Input: part model. Units: mm. Frame: model coordinates. Face numbers are marked on the shaded views. A direction names the side the tool comes from. Give positions to 0.01 mm unless a question says otherwise; leave off trailing zeros. Loops run counter-clockwise (first coordinate to the right, second up) from the corner with the lowest first, then second, coordinate; pieces in that order, holes last. Notation, with made-up numbers: (-34, 75) - (-7, 75) arc R21 ccw to (-7, 91) - close; hole circle Ø5 at (27.25, 63.5). An arc over 180 degrees is marked (long way). Answer as a JSON object with one key per item and string values. Group by question number.
(1) Access query for the marked faces 5, 6 and 7. Directions: +Z, -Z, +X, -X, +Y, -Y. A direction counts if a zero-diameter tool reaches every point of the face in a straight line with its end or side. Return the directions, or none.
(2) Section query D-D (x = -8). Return loops of the section in (y, z).
(3) Section query C-C (y = 8). Return loops of the section in (x, z).
(4) Pin query (flat end, axial travel): P1, Ø1, axis at x = -2, z = -16.5, coming from the +Y side; P2, Ø12, axis at x = 2.5, y = -5.5, coming from the +Z side; P3, Ø3, axis at x = -7.5, y = -1, coming from the +Z side; P4, Ø8, axis at x = -7, y = 4, coming from the -Z side. Return the tip coordinate at first contact, or that it passes through.
(5) Mould query, pull axis X, two halves, no side actions, for the marked faces 1, 2, 3 and 4. Classes: +X half, -X half, draft (parallel to the pull), parting line (faces both ways), or undercut.
(6) Section query A-A (z = -45.9). Return loops of the section in (x, y) (3 decimals).
(7) Section query B-B (x = 8). Return loops of the section in (y, z), plus the area to 3 significant figures.
(8) Material intervals for L1, parallel to Y at x = 5.25, z = -13.5; L2, parallel to X at y = -9.4, z = -45.9; L3, parallel to Z at x = 1, y = -10.5, sorted ascending.
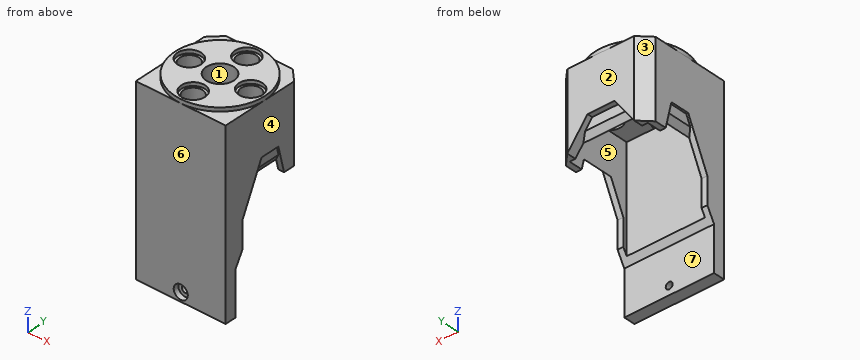
```python
from build123d import *

# Parameters (mm, degrees)
SKETCH_1_R                  = 11.7
EXTRUDE_1_DEPTH             = 7.7
SKETCH_1_3_R                = 2.5
CUT_EXTRUDE_1_DEPTH         = 19.250205478
SKETCH_1_5_R                = 3.1
SKETCH_1_5_R_2              = 2.5
CUT_EXTRUDE_2_DEPTH         = 0.9
CUT_EXTRUDE_START           = -6.8
SKETCH_1_6_R                = 3.1
SKETCH_1_6_R_2              = 2.5
CUT_EXTRUDE_3_DEPTH         = 0.9
EXTRUDE_START               = -7.7
SKETCH_2_W                  = 23.4
SKETCH_2_H                  = 2.4
SKETCH_2_H_2                = 4
EXTRUDE_3_DEPTH             = 40.5
SKETCH_3_W                  = 1.5
SKETCH_3_H                  = 23.4
EXTRUDE_4_DEPTH             = 40.3
EXTRUDE_START_2             = -1
EXTRUDE_5_DEPTH             = 6.7
CUT_EXTRUDE_5_DEPTH         = 55.842410596
CHAMFER_1_SIZE              = 3
CUT_EXTRUDE_6_REACH         = 56.842
EXTRUDE_6_REACH             = 52.961
EXTRUDE_6_DIRECTION_2_REACH = 52.961
EXTRUDE_7_REACH             = 52.961
EXTRUDE_7_DIRECTION_2_REACH = 52.961
HOLE_WIZARD_1_D             = 1.8
HOLE_WIZARD_1_CBORE_D       = 3.67
HOLE_WIZARD_1_CBORE_DEPTH   = 1.35
CUT_EXTRUDE_7_REACH         = 52.961
SKETCH_19_R                 = 3.6


with BuildPart() as part:
    # 草图1 → 凸台-拉伸1 (new body)
    with BuildSketch(Plane.XY):
        Circle(SKETCH_1_R)
    extrude(amount=-EXTRUDE_1_DEPTH)

    # 草图1<3> → 切除-拉伸1 (cut, through all)
    with BuildSketch(Plane.XY):
        with Locations((-8, 0)):
            Circle(SKETCH_1_3_R)
        with Locations((0, 8)):
            Circle(SKETCH_1_3_R)
        with Locations((8, 0)):
            Circle(SKETCH_1_3_R)
        with Locations((0, -8)):
            Circle(SKETCH_1_3_R)
    extrude(amount=-CUT_EXTRUDE_1_DEPTH, mode=Mode.SUBTRACT)

    # 草图1<5> → 切除-拉伸2 (cut)
    # profile 1 of 4: a face of its own
    with BuildSketch(Plane.XY):
        with Locations((-8, 0)):
            Circle(SKETCH_1_5_R)
        with Locations((-8, 0)):
            Circle(SKETCH_1_5_R_2, mode=Mode.SUBTRACT)
    # profile 2 of 4: a face of its own
    with BuildSketch(Plane.XY):
        with Locations((0, 8)):
            Circle(SKETCH_1_5_R)
        with Locations((0, 8)):
            Circle(SKETCH_1_5_R_2, mode=Mode.SUBTRACT)
    # profile 3 of 4: a face of its own
    with BuildSketch(Plane.XY):
        with Locations((8, 0)):
            Circle(SKETCH_1_5_R)
        with Locations((8, 0)):
            Circle(SKETCH_1_5_R_2, mode=Mode.SUBTRACT)
    # profile 4 of 4: a face of its own
    with BuildSketch(Plane.XY):
        with Locations((0, -8)):
            Circle(SKETCH_1_5_R)
        with Locations((0, -8)):
            Circle(SKETCH_1_5_R_2, mode=Mode.SUBTRACT)
    extrude(amount=-CUT_EXTRUDE_2_DEPTH, mode=Mode.SUBTRACT)

    # 草图1<6> → 切除-拉伸3 (cut)
    # profile 1 of 4: a face of its own
    with BuildSketch(Plane.XY.offset(CUT_EXTRUDE_START)):
        with Locations((-8, 0)):
            Circle(SKETCH_1_6_R)
        with Locations((-8, 0)):
            Circle(SKETCH_1_6_R_2, mode=Mode.SUBTRACT)
    # profile 2 of 4: a face of its own
    with BuildSketch(Plane.XY.offset(CUT_EXTRUDE_START)):
        with Locations((8, 0)):
            Circle(SKETCH_1_6_R)
        with Locations((8, 0)):
            Circle(SKETCH_1_6_R_2, mode=Mode.SUBTRACT)
    # profile 3 of 4: a face of its own
    with BuildSketch(Plane.XY.offset(CUT_EXTRUDE_START)):
        with Locations((0, -8)):
            Circle(SKETCH_1_6_R)
        with Locations((0, -8)):
            Circle(SKETCH_1_6_R_2, mode=Mode.SUBTRACT)
    # profile 4 of 4: a face of its own
    with BuildSketch(Plane.XY.offset(CUT_EXTRUDE_START)):
        with Locations((0, 8)):
            Circle(SKETCH_1_6_R)
        with Locations((0, 8)):
            Circle(SKETCH_1_6_R_2, mode=Mode.SUBTRACT)
    extrude(amount=-CUT_EXTRUDE_3_DEPTH, mode=Mode.SUBTRACT)

    # 草图2 → 凸台-拉伸3 (add)
    with BuildSketch(Plane.XY.offset(EXTRUDE_START)):
        with Locations((0, 10.5)):
            Rectangle(SKETCH_2_W, SKETCH_2_H)
        with Locations((0, -9.7)):
            Rectangle(SKETCH_2_W, SKETCH_2_H_2)
    extrude(amount=-EXTRUDE_3_DEPTH)

    # 草图3 → 凸台-拉伸4 (add)
    with BuildSketch(Plane.XY.offset(EXTRUDE_START)):
        with Locations((-10.95, 0)):
            Rectangle(SKETCH_3_W, SKETCH_3_H)
        with Locations((10.95, 0)):
            Rectangle(SKETCH_3_W, SKETCH_3_H)
    extrude(amount=-EXTRUDE_4_DEPTH)

    # 草图4 → 凸台-拉伸5 (add)
    with BuildSketch(Plane.XY.offset(EXTRUDE_START_2)):
        with BuildLine():
            Line((3.2e-08, 11.7), (-11.7, 11.7))
            Line((-11.7, 11.7), (-11.7, 0))
            ThreePointArc((-11.7, 0), (-8.273149328, 8.273149351), (3.2e-08, 11.7))
        make_face()
        with BuildLine():
            Line((11.7, 11.7), (3.2e-08, 11.7))
            ThreePointArc((3.2e-08, 11.7), (8.273149351, 8.273149328), (11.7, 0))
            Line((11.7, 0), (11.7, 11.7))
        make_face()
        with BuildLine():
            ThreePointArc((3e-09, -11.7), (-8.273149339, -8.273149341), (-11.7, 0))
            Line((-11.7, 0), (-11.7, -11.7))
            Line((-11.7, -11.7), (3e-09, -11.7))
        make_face()
        with BuildLine():
            Line((11.7, -11.7), (11.7, 0))
            ThreePointArc((11.7, 0), (8.273149341, -8.273149339), (3e-09, -11.7))
            Line((3e-09, -11.7), (11.7, -11.7))
        make_face()
    extrude(amount=-EXTRUDE_5_DEPTH)

    # 草图7 → 切除-拉伸5 (cut, through all)
    with BuildSketch(Plane.ZY.offset(11.7)):
        Polygon((-48.2, 11.7), (-48.2, -8.7), (-36.564101615, -8.7), (-33.1, -6.7), (-26.1, -6.7), (-14.1, -1), (-14.1, 4), (-21.1, 5.7), (-21.1, 11.7), align=None)
    extrude(amount=-CUT_EXTRUDE_5_DEPTH, mode=Mode.SUBTRACT)

    # 倒角1
    chamfer_1_edges = [part.edges().sort_by_distance(p)[0] for p in [
        (-11.7, 11.7, -11.05),
        (11.7, 11.7, -11.05),
    ]]
    chamfer(chamfer_1_edges, length=CHAMFER_1_SIZE)

    # 草图8 → 切除-拉伸6 (cut, up to next)
    with BuildSketch(Plane(origin=(0, 11.7, 0), x_dir=(1, 0, 0), z_dir=(0, 1, 0)), mode=Mode.PRIVATE) as cut_extrude_6_sk1:
        Polygon((8.7, 21.1), (3.414837489, 14.1), (-3.585162511, 14.1), (-8.7, 21.1), align=None)
    cut_extrude_6_tool1 = extrude(cut_extrude_6_sk1.sketch, amount=-CUT_EXTRUDE_6_REACH, mode=Mode.PRIVATE) & part.part
    add(cut_extrude_6_tool1.solids().sort_by_distance((-0.036531, 11.7, -18.097268))[0], mode=Mode.SUBTRACT)

    # 草图12 → 凸台-拉伸6 (add, up to next)
    with BuildSketch(Plane(origin=(0, 0, 0), x_dir=(0, 0, -1), z_dir=(1, 0, 0)), mode=Mode.PRIVATE) as extrude_6_sk1:
        Polygon((14.1, 10.3), (16.6, 10.3), (18.332050808, 9.3), (14.1, 9.3), align=None)
    extrude_6_tool1 = extrude(extrude_6_sk1.sketch, amount=EXTRUDE_6_REACH, mode=Mode.PRIVATE) - part.part
    add(extrude_6_tool1.solids().sort_by_distance((0, 9.757119, -15.820148))[0])

    # 草图12 → 凸台-拉伸6 direction 2 (add, up to next)
    with BuildSketch(Plane(origin=(0, 0, 0), x_dir=(0, 0, -1), z_dir=(1, 0, 0)), mode=Mode.PRIVATE) as extrude_6_direction_2_sk1:
        Polygon((14.1, 10.3), (16.6, 10.3), (18.332050808, 9.3), (14.1, 9.3), align=None)
    extrude_6_direction_2_tool1 = extrude(extrude_6_direction_2_sk1.sketch, amount=-EXTRUDE_6_DIRECTION_2_REACH, mode=Mode.PRIVATE) - part.part
    add(extrude_6_direction_2_tool1.solids().sort_by_distance((0, 9.757119, -15.820148))[0])

    # 草图13 → 凸台-拉伸7 (add, up to next)
    with BuildSketch(Plane(origin=(0, 0, 0), x_dir=(1, 0, 0), z_dir=(0, 1, 0)), mode=Mode.PRIVATE) as extrude_7_sk1:
        Polygon((10.2, 14.1), (11.2, 14.1), (11.2, 16.6), (10.2, 18.332050808), align=None)
    extrude_7_tool1 = extrude(extrude_7_sk1.sketch, amount=EXTRUDE_7_REACH, mode=Mode.PRIVATE) - part.part
    # 草图13 → 凸台-拉伸7 (add, up to next)
    with BuildSketch(Plane(origin=(0, 0, 0), x_dir=(1, 0, 0), z_dir=(0, 1, 0)), mode=Mode.PRIVATE) as extrude_7_sk2:
        Polygon((-10.2, 14.1), (-11.2, 14.1), (-11.2, 16.6), (-10.2, 18.332050808), align=None)
    extrude_7_tool2 = extrude(extrude_7_sk2.sketch, amount=EXTRUDE_7_REACH, mode=Mode.PRIVATE) - part.part
    add(extrude_7_tool1.solids().sort_by_distance((10.657119, 0, -15.820148))[0])
    add(extrude_7_tool2.solids().sort_by_distance((-10.657119, 0, -15.820148))[0])

    # 草图13 → 凸台-拉伸7 direction 2 (add, up to next)
    with BuildSketch(Plane(origin=(0, 0, 0), x_dir=(1, 0, 0), z_dir=(0, 1, 0)), mode=Mode.PRIVATE) as extrude_7_direction_2_sk1:
        Polygon((10.2, 14.1), (11.2, 14.1), (11.2, 16.6), (10.2, 18.332050808), align=None)
    extrude_7_direction_2_tool1 = extrude(extrude_7_direction_2_sk1.sketch, amount=-EXTRUDE_7_DIRECTION_2_REACH, mode=Mode.PRIVATE) - part.part
    # 草图13 → 凸台-拉伸7 direction 2 (add, up to next)
    with BuildSketch(Plane(origin=(0, 0, 0), x_dir=(1, 0, 0), z_dir=(0, 1, 0)), mode=Mode.PRIVATE) as extrude_7_direction_2_sk2:
        Polygon((-10.2, 14.1), (-11.2, 14.1), (-11.2, 16.6), (-10.2, 18.332050808), align=None)
    extrude_7_direction_2_tool2 = extrude(extrude_7_direction_2_sk2.sketch, amount=-EXTRUDE_7_DIRECTION_2_REACH, mode=Mode.PRIVATE) - part.part
    add(extrude_7_direction_2_tool1.solids().sort_by_distance((10.657119, 0, -15.820148))[0])
    add(extrude_7_direction_2_tool2.solids().sort_by_distance((-10.657119, 0, -15.820148))[0])

    # 孔1 (through all)
    with Locations(Plane(origin=(0, -11.7, -45.9), x_dir=(0, 0, -1), z_dir=(0, -1, 0))):
        with Locations((0, 0)):
            CounterBoreHole(HOLE_WIZARD_1_D / 2, HOLE_WIZARD_1_CBORE_D / 2, HOLE_WIZARD_1_CBORE_DEPTH)

    # 草图19 → 切除-拉伸7 (cut, up to next)
    with BuildSketch(Plane.XY, mode=Mode.PRIVATE) as cut_extrude_7_sk1:
        Circle(SKETCH_19_R)
    cut_extrude_7_tool1 = extrude(cut_extrude_7_sk1.sketch, amount=-CUT_EXTRUDE_7_REACH, mode=Mode.PRIVATE) & part.part
    add(cut_extrude_7_tool1.solids().sort_by_distance((0, 0, 0))[0], mode=Mode.SUBTRACT)


solid = part.part
```
Recorded:
{
 "1": {"face 5": "-Z", "face 6": "+Z, -Z, +X, -X, -Y", "face 7": "-Z, +X, -X, +Y"},
 "2": {"outline": "(-11.7, -48.2) - (-8.7, -48.2) - (-8.7, -36.56) - (-7.7, -34.83) - (-7.7, -7.7) - (-3.1, -7.7) - (-3.1, -6.8) - (-2.5, -6.8) - (-2.5, -0.9) - (-3.1, -0.9) - (-3.1, 0) - (-8.54, 0) - (-8.54, -1) - (-11.7, -1) - close; (2.5, -6.8) - (3.1, -6.8) - (3.1, -7.7) - (9.3, -7.7) - (9.3, -20.14) - (11.7, -20.14) - (11.7, -1) - (8.54, -1) - (8.54, 0) - (3.1, 0) - (3.1, -0.9) - (2.5, -0.9) - close"},
 "3": {"outline": "(-11.7, -21.1) - (-10.2, -21.1) - (-10.2, -7.7) - (-3.1, -7.7) - (-3.1, -6.8) - (-2.5, -6.8) - (-2.5, -0.9) - (-3.1, -0.9) - (-3.1, 0) - (-8.54, 0) - (-8.54, -1) - (-11.7, -1) - close; (2.5, -6.8) - (3.1, -6.8) - (3.1, -7.7) - (10.2, -7.7) - (10.2, -21.1) - (11.7, -21.1) - (11.7, -1) - (8.54, -1) - (8.54, 0) - (3.1, 0) - (3.1, -0.9) - (2.5, -0.9) - close"},
 "4": {"P1": "stops at y = 10.3", "P2": "stops at z = 0", "P3": "stops at z = -0.9", "P4": "stops at z = -21.1"},
 "5": {"face 1": "undercut", "face 2": "draft", "face 3": "-X half", "face 4": "+X half"},
 "6": {"outline": "(-11.7, -11.7) - (-1.835, -11.7) - (-1.835, -10.35) - (-0.9, -10.35) - (-0.9, -8.7) - (-11.7, -8.7) - close; (0.9, -10.35) - (1.835, -10.35) - (1.835, -11.7) - (11.7, -11.7) - (11.7, -8.7) - (0.9, -8.7) - close"},
 "7": {"outline": "(-11.7, -48.2) - (-8.7, -48.2) - (-8.7, -36.56) - (-7.7, -34.83) - (-7.7, -7.7) - (-3.1, -7.7) - (-3.1, -6.8) - (-2.5, -6.8) - (-2.5, -0.9) - (-3.1, -0.9) - (-3.1, 0) - (-8.54, 0) - (-8.54, -1) - (-11.7, -1) - close; (2.5, -6.8) - (3.1, -6.8) - (3.1, -7.7) - (9.3, -7.7) - (9.3, -20.17) - (11.7, -20.17) - (11.7, -1) - (8.54, -1) - (8.54, 0) - (3.1, 0) - (3.1, -0.9) - (2.5, -0.9) - close", "area": "313 mm^2"},
 "8": {"L1": "y = -11.7 to -7.7, 9.3 to 11.7", "L2": "x = -11.7 to -0.9, 0.9 to 11.7", "L3": "z = -48.2 to -47.44, -44.36 to -7.7, -6.8 to -0.9"}
}
